Here's how the part is built. I have some questions about the finished solid (model axes, mm). A direction names the side the tool comes from. Give positions to 0.01 mm unless a question says otherwise; leave off trailing zeros. Write each loop counter-clockwise with the first axis right and the second up, starting at its lowest first coordinate (ties: lowest second). Pieces come first, ordered by that corner, then holes. Notation, with made-up numbers: M 7,55 L 51,55 A28 ccw 51,80 Z; hole C -16.75,73 d11. An arc over 180 degrees is marked long. Use one line per item in the form item = value. Start each with the question number.
from build123d import *

# Parameters (mm, degrees)
BOSS_EXTRUDE1_DEPTH = 17
SKETCH2_W           = 70
SKETCH2_H           = 40
CUT_EXTRUDE1_DEPTH  = 7
CUT_EXTRUDE2_DEPTH  = 481.331856029


with BuildPart() as part:
    # Sketch1 → Boss-Extrude1 (new body)
    with BuildSketch(Plane(origin=(0, 0, 0), x_dir=(1, 0, 0), z_dir=(0, 1, 0))):
        Polygon((40, 489.668143971), (40, 269.668143971), (110, 269.668143971), (110, 490), (150, 490), (150, 10), (110, 10), (110, 229.668143971), (40, 229.668143971), (40, 9.668143971), (0, 9.668143971), (0, 489.668143971), align=None)
    extrude(amount=BOSS_EXTRUDE1_DEPTH)

    # Sketch2 → Cut-Extrude1 (cut)
    with BuildSketch(Plane(origin=(0, 17, 0), x_dir=(1, 0, 0), z_dir=(0, 1, 0))):
        with Locations((75, 249.668143971)):
            Rectangle(SKETCH2_W, SKETCH2_H)
    extrude(amount=-CUT_EXTRUDE1_DEPTH, mode=Mode.SUBTRACT)

    # Sketch3 → Cut-Extrude2 (cut, through all)
    with BuildSketch(Plane.XY.offset(-9.668143971)):
        Polygon((17.25, 0), (17.25, 7.25), (9.75, 7.25), (9.75, 10.25), (30.25, 10.25), (30.25, 7.25), (22.75, 7.25), (22.75, 0), align=None)
    cut_extrude2 = extrude(amount=-CUT_EXTRUDE2_DEPTH, mode=Mode.SUBTRACT)

    # Mirror1: Cut-Extrude2 across plane
    add(cut_extrude2.mirror(Plane(origin=(75, 0, 0), x_dir=(0, 0, 1), z_dir=(1, 0, 0))), mode=Mode.SUBTRACT)


solid = part.part
1) Thinking about a two-plate mould opening in Y: for faces 1 (the face through (20, 10.25, -246)), 2 (the face through (20, 12, -489.668)), 3 (the face through (130, 17, -253)), 4 (the face through (9, 0, -253)), which applies, released by +Y, released by -Y, zero draft, split by the parting line, or undercut?
2) Suppose I cut it at A-A, the plane y = 4. List the corners of the cut face in (x, z) for me, and give its area (3 significant figures).
3) Will these pins go through, and if not, where does the flat tip stop? P1, Ø3, axis at x = 79.5, y = 6, coming from the -Z side; P2, Ø20, axis at x = 80.5, z = -241, coming from the +Y side; P3, Ø8.5, axis at x = 22.5, y = 9, coming from the -Z side.
4) Suppose I cut it at C-C, the plane x = 61. List the corners of the cut face in (y, z) for me, and give its area (3 significant figures).
5) Please list where these lines run through material, in increasing order: line 1 (X direction, y = 5, z = -52.5); line 2 (X direction, y = 2.5, z = -230.5); line 3 (X direction, y = 8, z = -179.5).
6) Suppose I cut it at B-B, the plane z = -279.5. List the corners of the cut face in (x, y) for me, and give its area (3 significant figures).
7) On a 3-axis mill with a long thin cutter (end or side, diameter ignored), from which of +Z, -Z, +X, -X, +Y, -Y can I reach the whole of each face in a straight line? I mean faces 5 (the face through (75, 5, -229.668)), 6 (the face through (75, 10, -250)), 7 (the face through (130, 12, -10)), 8 (the face through (130, 10.25, -247)), 9 (the face through (75, 5, -269.668)). Say none if no direction works.
Checks:
q1.face_1 = undercut
q1.face_2 = zero draft
q1.face_3 = released by +Y
q1.face_4 = released by -Y
q2.outline = M 0,-489.67 L 17.25,-489.67 L 17.25,-9.67 L 0,-9.67 Z; M 22.75,-489.67 L 40,-489.67 L 40,-269.67 L 110,-269.67 L 110,-490 L 127.25,-490 L 127.25,-10 L 110,-10 L 110,-229.67 L 40,-229.67 L 40,-9.67 L 22.75,-9.67 Z; M 132.75,-490 L 150,-490 L 150,-10 L 132.75,-10 Z
q2.area = 35,900 mm^2
q3.P1 = -269.67
q3.P2 = 10
q3.P3 = -489.67
q4.outline = M 0,-269.67 L 10,-269.67 L 10,-229.67 L 0,-229.67 Z
q4.area = 400 mm^2
q5.line_1 = 0 to 17.25, 22.75 to 40, 110 to 127.25, 132.75 to 150
q5.line_2 = 0 to 17.25, 22.75 to 127.25, 132.75 to 150
q5.line_3 = 0 to 9.75, 30.25 to 40, 110 to 119.75, 140.25 to 150
q6.outline = M 0,0 L 17.25,0 L 17.25,7.25 L 9.75,7.25 L 9.75,10.25 L 30.25,10.25 L 30.25,7.25 L 22.75,7.25 L 22.75,0 L 40,0 L 40,17 L 0,17 Z; M 110,0 L 127.25,0 L 127.25,7.25 L 119.75,7.25 L 119.75,10.25 L 140.25,10.25 L 140.25,7.25 L 132.75,7.25 L 132.75,0 L 150,0 L 150,17 L 110,17 Z
q6.area = 1,160 mm^2
q7.face_5 = +Z, +Y, -Y
q7.face_6 = +Z, -Z, +Y
q7.face_7 = +Z, +X, +Y, -Y
q7.face_8 = +Z, -Z
q7.face_9 = -Z, +Y, -Y
